Geometry check sheet. Reference: the model listing, model coordinates, mm. Give positions to 0.01 mm unless a question says otherwise; leave off trailing zeros. Loops run counter-clockwise (first coordinate to the right, second up) from the corner with the lowest first, then second, coordinate; pieces in that order, holes last. Notation, with made-up numbers: (-14.75, 28.5) -> (-7.75, 28.5) arc R20 cw to (-7.75, 36.5) -> close; hole circle Ø8 at (-13, -7). An arc over 180 degrees is marked (long way). Write item = value, one per line.
```python
from build123d import *

# Parameters (mm, degrees)
BOSS_EXTRUDE1_DEPTH         = 1.5875
F_10_CLEARANCE_HOLE1_D      = 4.9784
F_1_4_0_25_DIAMETER_HOLE1_D = 6.35
F_1_4_0_25_DIAMETER_HOLE2_D = 6.35


with BuildPart() as part:
    # Sketch1 → Boss-Extrude1 (new body)
    with BuildSketch(Plane.XY):
        Polygon((233.807000506, -12.7), (233.807000506, -65.7225), (342.900001016, -65.7225), (342.900001016, -12.7), (317.500001016, 12.7), (259.207000506, 12.7), align=None)
    extrude(amount=BOSS_EXTRUDE1_DEPTH)

    # #10 Clearance Hole1 (through all)
    with Locations(Plane(origin=(0, 0, 0), x_dir=(-1, 0, 0), z_dir=(0, 0, -1))):
        with Locations((-330.199999492, -12.7), (-304.799999492, 0), (-279.399999492, 0), (-252.857001004, -8e-09)):
            Hole(F_10_CLEARANCE_HOLE1_D / 2)

    # 1/4 (0.25) Diameter Hole1 (through all)
    with Locations(Plane(origin=(0, 0, 0), x_dir=(-1, 0, 0), z_dir=(0, 0, -1))):
        with Locations((-330.200001016, -61.9125)):
            Hole(F_1_4_0_25_DIAMETER_HOLE1_D / 2)

    # 1/4 (0.25) Diameter Hole2 (through all)
    with Locations(Plane.XY.offset(1.5875)):
        with Locations((299.085001016, -24.525188452), (241.935001016, -52.465188452)):
            Hole(F_1_4_0_25_DIAMETER_HOLE2_D / 2)


solid = part.part
```
Item 1: Section check C-C, the plane y = 0. Record the cut outline in (x, z).
Answer:
outline = (246.51, 0) -> (250.37, 0) -> (250.37, 1.59) -> (246.51, 1.59) -> close; (255.35, 0) -> (276.91, 0) -> (276.91, 1.59) -> (255.35, 1.59) -> close; (281.89, 0) -> (302.31, 0) -> (302.31, 1.59) -> (281.89, 1.59) -> close; (307.29, 0) -> (330.2, 0) -> (330.2, 1.59) -> (307.29, 1.59) -> close
Item 2: Section check B-B, the plane x = 304.8. Record the cut outline in (y, z), plus the area to 3 significant figures.
Answer:
outline = (-65.72, 0) -> (-2.49, 0) -> (-2.49, 1.59) -> (-65.72, 1.59) -> close; (2.49, 0) -> (12.7, 0) -> (12.7, 1.59) -> (2.49, 1.59) -> close
area = 117 mm^2
Item 3: Section check A-A, the plane x = 330.2. Record the cut outline in (y, z).
Answer:
outline = (-65.72, 0) -> (-65.09, 0) -> (-65.09, 1.59) -> (-65.72, 1.59) -> close; (-58.74, 0) -> (-15.19, 0) -> (-15.19, 1.59) -> (-58.74, 1.59) -> close; (-10.21, 0) -> (0, 0) -> (0, 1.59) -> (-10.21, 1.59) -> close
Item 4: Thickness scan on L1, parallel to Y at x = 279.4, z = 0.55; L2, parallel to Y at x = 331.5, z = 0.8; L3, parallel to Y at x = 281, z = 0.5. Record the ranges inside material, lowest first. Write a range as [from, to].
Answer:
L1 = [-65.72, -2.49], [2.49, 12.7]
L2 = [-65.72, -64.81], [-59.02, -14.82], [-10.58, -1.3]
L3 = [-65.72, -1.91], [1.91, 12.7]
Item 5: Gauge pin test, flat ends, axial feed: pin 1 (5.5 mm diameter, centred on x = 304.8, y = 0, fed in from +Z); pin 2 (5 mm diameter, centred on x = 241.94, y = -52.47, fed in from -Z). Record the tip position at first contact, or that the pin passes through.
Answer:
pin_1 = 1.59
pin_2 = through
Item 6: Draft check along Y on faces 1 (the flat face through (288, -26, 0)), 2 (the flat face through (246.685, 0.178, 0.783)), 3 (the cylindrical face through (250.37, 0.11, 0.8)). Enter one of: +Y half, -Y half, draft (parallel to the pull), parting line (faces both ways), or undercut.
Answer:
face_1 = draft
face_2 = +Y half
face_3 = undercut
Item 7: Section check D-D, the plane z = 0.25. Give the number of separate pieces and of enclosed holes in the cut face, plus the area to 3 significant figures.
Answer:
separate_pieces = 1
enclosed_holes = 7
area = 7,740 mm^2
